Here's how the part is built. I have some questions about the finished solid (model axes, mm). A direction names the side the tool comes from. Round coordinates to 2 decimals unless told otherwise and drop trailing zeros. Write each loop counter-clockwise with the first axis right and the second up, starting at its lowest first coordinate (ties: lowest second). Pieces come first, ordered by that corner, then holes. Notation, with made-up numbers: (-14.5, -25) -> (-5.5, -25) arc R28 cw to (-5.5, 4) -> close; hole circle Ø7 at (51.25, 26.25). An arc over 180 degrees is marked (long way). Put each result on its own line as item: value. Start each with the question number.
1. Suppose I cut it at A-A (z = 12.5). Count the separate pieces of the cut face and the enclosed holes in it, then the cut area to 3 significant figures.
2. Suppose I cut it at B-B (x = 3.5). Please give me the cut outline in (y, z), then the cut area to 3 significant figures.
3. We'd pull the mould along X, two halves only. Please class faces 1 (the face through (-12, -2, 9)), 2 (the face through (14.92, -11.41, 1.48)), 3 (the face through (6, -4, 13)), 4 (the face through (0, 10, 12)): +X half, -X half, draft (parallel to the pull), parting line (faces both ways), or undercut.
4. Suppose I cut it at C-C (y = -0.75). Please give me the cut outline in (x, z), then the cut area to 3 significant figures.
5. For pin 1 (5.5 mm diameter, centred on x = 0, z = 12, fed in from -Y); pin 2 (2 mm diameter, centred on x = 11, z = 6, fed in from +Y); pin 3 (0.8 mm diameter, centred on x = 7, y = -5, fed in from -Z), each with a flat end and sliding along its axis, tell me the tip position at first contact or that it passes through.
6. I need wall thicknesses on probe 1 along X at (y, z) = (-2, 16.5); probe 2 along Y at (x, z) = (3.5, 4); probe 3 along Y at (x, z) = (-0.5, 4.75). Which ranges of each line are inside material? Lowest first, please. Write a range as from..to.
7. Which directions (+Z, -Z, +X, -X, +Y, -Y) give clear straight access to the entire face, cutting with the end or side of a thin tool? Please do faces 5 (the face through (-7, -2.041, 11)), 6 (the face through (0, 11.707, 1)), 7 (the face through (12.021, 5.232, 12.367)).
8. Suppose I cut it at D-D (z = 18.5). Please give me the cut outline in (x, y), then the cut area to 3 significant figures.
```python
from build123d import *

# Parameters (mm, degrees)
EXTRUDE_1_DEPTH     = 3
EXTRUDE_2_DEPTH     = 19
CUT_EXTRUDE_1_DEPTH = 17.5
SKETCH_4_W          = 2
SKETCH_4_H          = 4
EXTRUDE_3_DEPTH     = 12.5
EXTRUDE_4_DEPTH     = 4
CUT_EXTRUDE_2_DEPTH = 4


with BuildPart() as part:
    # 草图1 → 凸台-拉伸1 (new body)
    with BuildSketch(Plane.XY):
        with BuildLine():
            Line((-14.207106781, 11.707106781), (14.207106781, 11.707106781))
            ThreePointArc((14.207106781, 11.707106781), (14.914213562, 11.414213562), (15.207106781, 10.707106781))
            Line((15.207106781, 10.707106781), (15.207106781, -10.707106781))
            ThreePointArc((15.207106781, -10.707106781), (14.914213562, -11.414213562), (14.207106781, -11.707106781))
            Line((14.207106781, -11.707106781), (-14.207106781, -11.707106781))
            ThreePointArc((-14.207106781, -11.707106781), (-14.914213562, -11.414213562), (-15.207106781, -10.707106781))
            Line((-15.207106781, -10.707106781), (-15.207106781, 10.707106781))
            ThreePointArc((-15.207106781, 10.707106781), (-14.914213562, 11.414213562), (-14.207106781, 11.707106781))
        make_face()
    extrude(amount=EXTRUDE_1_DEPTH)

    # 草图2 → 凸台-拉伸2 (add)
    with BuildSketch(Plane.XY.offset(3)):
        with BuildLine():
            Line((-10.5, 10), (-10.5, 6.5))
            Line((-10.5, 6.5), (-13.5, 4))
            Line((-13.5, 4), (-13.5, -8.5))
            ThreePointArc((-13.5, -8.5), (-13.060660172, -9.560660172), (-12, -10))
            Line((-12, -10), (12, -10))
            ThreePointArc((12, -10), (13.060660172, -9.560660172), (13.5, -8.5))
            Line((13.5, -8.5), (13.5, 4))
            Line((13.5, 4), (10.5, 6.5))
            Line((10.5, 6.5), (10.5, 10))
            Line((10.5, 10), (-10.5, 10))
        make_face()
    extrude(amount=EXTRUDE_2_DEPTH)

    # 草图3 → 切除-拉伸1 (cut)
    with BuildSketch(Plane(origin=(0, 0, 0), x_dir=(-1, 0, 0), z_dir=(0, 0, -1))):
        with BuildLine():
            Line((12, -6.525638569), (12, 1.761252493))
            ThreePointArc((12, 1.761252493), (11.959963562, 1.957297186), (11.846265914, 2.121946154))
            Line((11.846265914, 2.121946154), (5.89511077, 7.835055092))
            ThreePointArc((5.89511077, 7.835055092), (5.735463679, 7.938229317), (5.548844856, 7.974361431))
            Line((5.548844856, 7.974361431), (-5.548844856, 7.974361431))
            ThreePointArc((-5.548844856, 7.974361431), (-5.735463679, 7.938229317), (-5.89511077, 7.835055092))
            Line((-5.89511077, 7.835055092), (-11.846265914, 2.121946154))
            ThreePointArc((-11.846265914, 2.121946154), (-11.959963562, 1.957297186), (-12, 1.761252493))
            Line((-12, 1.761252493), (-12, -6.525638569))
            ThreePointArc((-12, -6.525638569), (-11.560660172, -7.58629874), (-10.5, -8.025638569))
            Line((-10.5, -8.025638569), (10.5, -8.025638569))
            ThreePointArc((10.5, -8.025638569), (11.560660172, -7.58629874), (12, -6.525638569))
        make_face()
    extrude(amount=-CUT_EXTRUDE_1_DEPTH, mode=Mode.SUBTRACT)

    # 草图4 → 凸台-拉伸3 (add)
    with BuildSketch(Plane(origin=(0, 0, 17.5), x_dir=(-1, 0, 0), z_dir=(0, 0, -1))):
        with Locations((-7, -4.041451884)):
            Rectangle(SKETCH_4_W, SKETCH_4_H)
        with Locations((0, 3.099976544)):
            Rectangle(SKETCH_4_W, SKETCH_4_H)
        with Locations((7, -4.041451884)):
            Rectangle(SKETCH_4_W, SKETCH_4_H)
    extrude(amount=EXTRUDE_3_DEPTH)

    # 草图5 → 凸台-拉伸4 (add)
    with BuildSketch(Plane.XZ.offset(-1.099976544)):
        Polygon((1, 5), (-1, 5), (-0.5, 2.5), (0.5, 2.5), align=None)
    extrude(amount=-EXTRUDE_4_DEPTH)

    # 草图6 → 切除-拉伸2 (cut)
    with BuildSketch(Plane.XZ.offset(6.041451884)):
        Polygon((8, 5), (8, 7.5), (7.5, 5), align=None)
        Polygon((6.5, 5), (6, 5), (6, 7.5), align=None)
        Polygon((-6, 5), (-6, 7.5), (-6.5, 5), align=None)
        Polygon((-7.5, 5), (-8, 5), (-8, 7.5), align=None)
    extrude(amount=-CUT_EXTRUDE_2_DEPTH, mode=Mode.SUBTRACT)


solid = part.part
```
Verdict:
1. separate pieces: 4
1. enclosed holes: 1
1. area: 189 mm^2
2. outline: (-11.71, 0) -> (-8.03, 0) -> (-8.03, 17.5) -> (7.97, 17.5) -> (7.97, 0) -> (11.71, 0) -> (11.71, 3) -> (10, 3) -> (10, 22) -> (-10, 22) -> (-10, 3) -> (-11.71, 3) -> close
2. area: 170 mm^2
3. face 1: undercut
3. face 2: +X half
3. face 3: undercut
3. face 4: draft
4. outline: (-15.21, 0) -> (-12, 0) -> (-12, 17.5) -> (12, 17.5) -> (12, 0) -> (15.21, 0) -> (15.21, 3) -> (13.5, 3) -> (13.5, 22) -> (-13.5, 22) -> (-13.5, 3) -> (-15.21, 3) -> close
4. area: 184 mm^2
5. pin 1: stops at y = -10
5. pin 2: stops at y = 10
5. pin 3: stops at z = 5
6. probe 1: x = -13.5..-12, 12..13.5
6. probe 2: y = -10..-8.03, 7.97..10
6. probe 3: y = -10..-8.03, 1.1..5.1, 7.97..10
7. face 5: -Z
7. face 6: +Z, -Z, +X, -X, +Y
7. face 7: +Z, +X, +Y
8. outline: (-13.5, -8.5) arc R1.5 ccw to (-12, -10) -> (12, -10) arc R1.5 ccw to (13.5, -8.5) -> (13.5, 4) -> (10.5, 6.5) -> (10.5, 10) -> (-10.5, 10) -> (-10.5, 6.5) -> (-13.5, 4) -> close
8. area: 511 mm^2
